from build123d import *

# Parameters (mm, degrees)
SKETCH1_W          = 40
SKETCH1_H          = 130
SKETCH1_R          = 6.35
SKETCH1_R_2        = 3.175
BASE_FLANGE1_DEPTH = 6.35
EDGE_FLANGE1_DEPTH = 40
EDGE_FLANGE2_DEPTH = 40
SKETCH20_R         = 3.175
CUT_EXTRUDE3_DEPTH = 6.35


# Sheet-metal steps are written as plain solids
with BuildPart() as part:
    # Sketch1 → Base-Flange1 (new body)
    with BuildSketch(Plane(origin=(0, 0, 0), x_dir=(0, 0, -1), z_dir=(1, 0, 0))):
        with Locations((20, -65)):
            Rectangle(SKETCH1_W, SKETCH1_H)
        with Locations((20, -20)):
            Circle(SKETCH1_R, mode=Mode.SUBTRACT)
        with Locations((20, -64.45)):
            Circle(SKETCH1_R_2, mode=Mode.SUBTRACT)
    extrude(amount=-BASE_FLANGE1_DEPTH)

    # Edge-Flange1 section (across the edge) → Edge-Flange1 (add)
    with BuildSketch(Plane(origin=(0, -130.268100475, 0), x_dir=(0.7660444431189817, 0.642787609686535, 0), z_dir=(0, 0, -1))):
        with BuildLine():
            Line((-6.35, 0.268100475), (-6.35, 25))
            Line((-6.35, 25), (0, 25))
            Line((0, 25), (0, 0.268100475))
            ThreePointArc((0, 0.268100475), (0.044422416, 0.016168437), (0.172331663, -0.205376879))
            Line((0.172331663, -0.205376879), (-4.692050551, -4.2870782))
            ThreePointArc((-4.692050551, -4.2870782), (-5.922625726, -2.155659473), (-6.35, 0.268100475))
        make_face()
    extrude(amount=EDGE_FLANGE1_DEPTH)

    # Edge-Flange2 section (across the edge) → Edge-Flange2 (add)
    with BuildSketch(Plane(origin=(11.377639692, -153.706289753, -40), x_dir=(-1, 0, 0), z_dir=(0, 0, 1))):
        with BuildLine():
            Line((-6.35, 0.268100475), (-6.35, 30))
            Line((-6.35, 30), (0, 30))
            Line((0, 30), (0, 0.268100475))
            ThreePointArc((0, 0.268100475), (0.044422416, 0.016168437), (0.172331663, -0.205376879))
            Line((0.172331663, -0.205376879), (-4.692050551, -4.2870782))
            ThreePointArc((-4.692050551, -4.2870782), (-5.922625726, -2.155659473), (-6.35, 0.268100475))
        make_face()
    extrude(amount=EDGE_FLANGE2_DEPTH)

    # Sketch20 → Cut-Extrude3 (cut)
    with BuildSketch(Plane(origin=(17.727639692, 0, 0), x_dir=(0, 0, -1), z_dir=(1, 0, 0))):
        with Locations(Location((10, -168.84033999, 0), (0, 0, 90))):
            Circle(SKETCH20_R)
    extrude(amount=-CUT_EXTRUDE3_DEPTH, mode=Mode.SUBTRACT)


solid = part.part
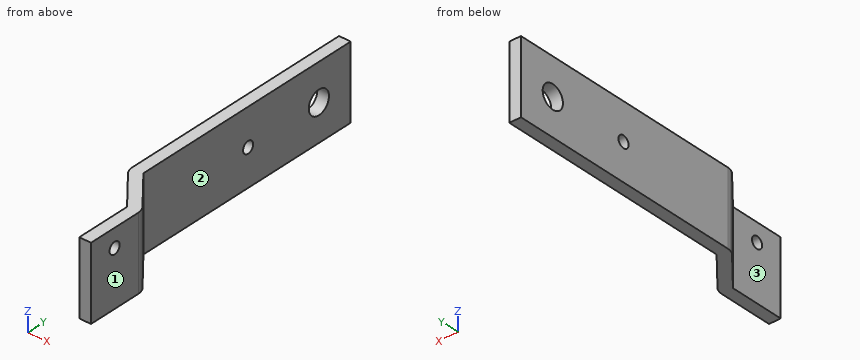
Part model, mm, in its own coordinate system. Face numbers are marked on the shaded views. A direction names the side the tool comes from. Round coordinates to 2 decimals unless told otherwise and drop trailing zeros. Loops run counter-clockwise (first coordinate to the right, second up) from the corner with the lowest first, then second, coordinate; pieces in that order, holes last. Notation, with made-up numbers: (12.5, -1) - (54.5, -1) arc R24 ccw to (54.5, 10) - close; hole circle Ø1 at (67, -1.5). An arc over 180 degrees is marked (long way). Answer as a JSON object with one key per item and string values.
Item 1: Pin check, flat tips, straight feed: pin 1 (11.5 mm diameter, centred on y = -20, z = -20, fed in from -X); pin 2 (12 mm diameter, centred on x = 7, z = -28.5, fed in from +Y); pin 3 (15 mm diameter, centred on y = -172, z = -26.5, fed in from -X). Stop position of each tip, or through.
Output:
{"pin 1": "through", "pin 2": "y = -131.46", "pin 3": "x = 11.38"}
Item 2: Wall check: L1, parallel to Y at x = -3.25, z = -20 (3 decimals); L2, parallel to Y at x = -1.5, z = -20 (3 decimals); L3, parallel to X at y = -99.5, z = -4. Give the ranges that are in metal, low to high.
Output:
{"L1": "-136.274 to -67.625, -61.275 to -26.35, -13.65 to 0", "L2": "-138.359 to -67.625, -61.275 to -26.35, -13.65 to 0", "L3": "-6.35 to 0"}
Item 3: Band-saw the part on C-C on z = -10. List the corners of the cut face in (x, y).
Output:
{"outline": "(-6.35, -130) arc R7.09 ccw to (-4.69, -134.56) - (11.21, -153.5) arc R0.74 cw to (11.38, -153.97) - (11.38, -165.67) - (17.73, -165.67) - (17.73, -153.97) arc R7.09 ccw to (16.07, -149.42) - (0.17, -130.47) arc R0.74 cw to (0, -130) - (0, 0) - (-6.35, 0) - close; (11.38, -183.71) - (17.73, -183.71) - (17.73, -172.02) - (11.38, -172.02) - close"}
Item 4: Band-saw the part on D-D on z = -34. List the corners of the cut face in (x, y).
Output:
{"outline": "(-6.35, -130) arc R7.09 ccw to (-4.69, -134.56) - (11.21, -153.5) arc R0.74 cw to (11.38, -153.97) - (11.38, -183.71) - (17.73, -183.71) - (17.73, -153.97) arc R7.09 ccw to (16.07, -149.42) - (0.17, -130.47) arc R0.74 cw to (0, -130) - (0, 0) - (-6.35, 0) - close"}
Item 5: Band-saw the part on A-A on y = -64.45. List the corners of the cut face in (x, z) (3 decimals).
Output:
{"outline": "(-6.35, -40) - (0, -40) - (0, -23.175) - (-6.35, -23.175) - close; (-6.35, -16.825) - (0, -16.825) - (0, 0) - (-6.35, 0) - close"}
Item 6: Band-saw the part on B-B on z = -20. List the corners of the cut face in (x, y) (3 decimals).
Output:
{"outline": "(-6.35, -130) arc R7.087 ccw to (-4.692, -134.555) - (11.205, -153.501) arc R0.737 cw to (11.378, -153.974) - (11.378, -183.706) - (17.728, -183.706) - (17.728, -153.974) arc R7.087 ccw to (16.07, -149.419) - (0.172, -130.473) arc R0.737 cw to (0, -130) - (0, -67.625) - (-6.35, -67.625) - close; (-6.35, -61.275) - (0, -61.275) - (0, -26.35) - (-6.35, -26.35) - close; (-6.35, -13.65) - (0, -13.65) - (0, 0) - (-6.35, 0) - close"}
Item 7: Tool access for the marked faces 1, 2 and 3: list every direction of +Z, -Z, +X, -X, +Y, -Y with a clear straight run to the whole face (end or side of a thin tool).
Output:
{"face 1": "+Z, -Z, +X, +Y, -Y", "face 2": "+Z, -Z, +X, +Y", "face 3": "+Z, -Z, -X, -Y"}
